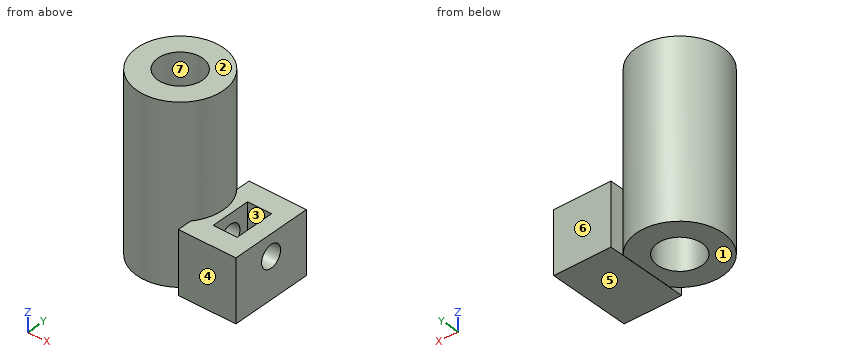
from build123d import *

# Parameters (mm, degrees)
CYLINDER005_R     = 1.6
CYLINDER005_DEPTH = 22.9
CYLINDER003_R     = 3.2
CYLINDER003_DEPTH = 50
CUBE003_W         = 3.45
CUBE003_H         = 5.8
CUBE003_DEPTH     = 11.11
CUBE002_W         = 8.25
CUBE002_H         = 11.91
CUBE002_DEPTH     = 8.91
CYLINDER004_R     = 6.2
CYLINDER004_DEPTH = 25


with BuildPart() as cylinder005:
    # cylinder005 → cylinder005 (new body)
    with BuildSketch(Plane(origin=(0, 0, 5.83), x_dir=(0, 0, -1), z_dir=(1, 0, 0))):
        Circle(CYLINDER005_R)
    extrude(amount=CYLINDER005_DEPTH)


with BuildPart() as union002:
    # cylinder003 → cylinder003 (new body)
    with BuildSketch(Plane.XY.offset(-1)):
        Circle(CYLINDER003_R)
    extrude(amount=CYLINDER003_DEPTH)

    # union002: union cylinder005
    add(cylinder005.part)


with BuildPart() as cube003:
    # cube003 → cube003 (new body)
    with BuildSketch(Plane(origin=(-1.725, -2.9, -3.6), x_dir=(1, 0, 0), z_dir=(0, 0, 1))):
        with Locations((1.725, 2.9)):
            Rectangle(CUBE003_W, CUBE003_H)
    extrude(amount=CUBE003_DEPTH)


with BuildPart() as difference002:
    # cube002 → cube002 (new body)
    with BuildSketch(Plane(origin=(-4.125, -5.955, -6.455), x_dir=(1, 0, 0), z_dir=(0, 0, 1))):
        with Locations((4.125, 5.955)):
            Rectangle(CUBE002_W, CUBE002_H)
    extrude(amount=CUBE002_DEPTH)

    # difference002: cut cube003
    add(cube003.part, mode=Mode.SUBTRACT)


with BuildPart() as difference002_1:
    # difference002 placement: moved
    add(difference002.part.moved(Location((8.95, 0, 6.425))))


with BuildPart() as wheel_fit_holder:
    # cylinder004 → cylinder004 (new body)
    with BuildSketch(Plane.XY):
        Circle(CYLINDER004_R)
    extrude(amount=CYLINDER004_DEPTH)

    # union003: union difference002
    add(difference002_1.part)

    # difference003: cut union002
    add(union002.part, mode=Mode.SUBTRACT)


solid = wheel_fit_holder.part
The listing builds one solid part. Answer for the finished solid, in the listing's coordinates (mm). Face numbers are marked on the shaded views. A direction names the side the tool comes from. Give positions to 0.01 mm unless a question says otherwise; leave off trailing zeros. Write each loop counter-clockwise with the first axis right and the second up, starting at its lowest first coordinate (ties: lowest second). Pieces come first, ordered by that corner, then holes.
1) A tool of negligible diameter and unlimited length cuts with its end or side. For the marked faces 1, 2, 3 and 4, from which of +Z, -Z, +X, -X, +Y, -Y can it reach the whole face along a straight path? Write none if from no direction.
2) Section A-A (y = 0) is taken. Write down the section's boundary in (x, z) (3 decimals), and give its area (3 significant figures).
3) For a pull along Y with two mould halves and no side action, classify the marked faces 5, 6 and 7 as pulls with the +Y half, pulls with the -Y half, needs draft (parallel to the pull), parting line crosses it, or undercut.
4) Section B-B (x = 0) is taken. Write down the section's boundary in (y, z).
5) Section D-D (z = 9.5) is taken. Write down the section's boundary in (x, y), and give its area (3 significant figures).
6) Given P1, Ø1.7, axis at x = 9, y = 1, coming from the +Z side (3 decimals); P2, Ø1, axis at y = 4, z = 14, coming from the -X side; P3, Ø4, axis at x = 8, z = 2, coming from the +Y side (3 decimals), each flat-ended and moving along its own axis, determine where each tip first touches the part or whether it passes through.
7) Find the intervals of material crossed by L1, parallel to Y at x = 5.5, z = 5.83 (3 decimals); L2, parallel to X at y = 0, z = 14.5; L3, parallel to Z at x = 4.5, y = 0, in increasing order.
Response:
1. face 1: -Z, -X, +Y, -Y
1. face 2: +Z, +X, -X, +Y, -Y
1. face 3: +Z
1. face 4: +Z, -Z, +X, -Y
2. outline: (-6.2, 0) - (-3.2, 0) - (-3.2, 25) - (-6.2, 25) - close; (3.2, 0) - (4.825, 0) - (4.825, -0.03) - (13.075, -0.03) - (13.075, 4.23) - (10.675, 4.23) - (10.675, 2.825) - (7.225, 2.825) - (7.225, 4.23) - (3.2, 4.23) - close; (3.2, 7.43) - (7.225, 7.43) - (7.225, 8.88) - (6.2, 8.88) - (6.2, 25) - (3.2, 25) - close; (10.675, 7.43) - (13.075, 7.43) - (13.075, 8.88) - (10.675, 8.88) - close
2. area: 170 mm2
3. face 5: needs draft
3. face 6: pulls with the +Y half
3. face 7: undercut
4. outline: (-6.2, 0) - (-3.2, 0) - (-3.2, 25) - (-6.2, 25) - close; (3.2, 0) - (6.2, 0) - (6.2, 25) - (3.2, 25) - close
5. outline: circle Ø12.4 at (0, 0); hole circle Ø6.4 at (0, 0)
5. area: 88.6 mm2
6. P1: stops at z = 2.825
6. P2: stops at x = -5.12
6. P3: stops at y = 5.955
7. L1: y = -5.955 to -1.6, 1.6 to 5.955
7. L2: x = -6.2 to -3.2, 3.2 to 6.2
7. L3: z = 0 to 4.23, 7.43 to 25
